Check sheet for the modelled part. Datum: model origin and axes. Units: mm. Face numbers are marked on the shaded views. A direction names the side the tool comes from. Round coordinates to 2 decimals unless told otherwise and drop trailing zeros. Write each loop counter-clockwise with the first axis right and the second up, starting at its lowest first coordinate (ties: lowest second). Pieces come first, ordered by that corner, then holes. Notation, with made-up numbers: (22.25, 81) - (79.25, 81) arc R9 cw to (79.25, 85) - close; hole circle Ø7 at (-29.75, 13). An arc over 180 degrees is marked (long way). Use one line per item in the form item = value. Start each with the question number.
1) Section check C-C (z = 8). Record the boundary of the cut face in (x, y), then the cut area to 3 significant figures.
2) Section check A-A (x = -32.5). Record the boundary of the cut face in (y, z).
3) Set-up check for the marked faces 1, 2 and 3: record each of +Z, -Z, +X, -X, +Y, -Y from which the full face is reachable in a straight line by a thin tool's end or side.
4) Gauge pin test, flat ends, axial feed: P1, Ø4.5, axis at x = 29.5, z = -2.5, coming from the +Y side; P2, Ø14, axis at y = 22, z = 2, coming from the +X side; P3, Ø6, axis at x = -32.5, z = 0, coming from the +Y side; P4, Ø7, axis at y = 2.5, z = -3, coming from the -X side. Record the tip position at first contact, or that the pin passes through.
5) Draft check along X on the marked faces 4, 5 and 6. Enter one of: +X half, -X half, draft (parallel to the pull), parting line (faces both ways), or undercut.
6) Section check B-B (y = 0). Record the boundary of the cut face in (x, z).
7) Scan lines: probe 1 along X at (y, z) = (22, -1.25); probe 2 along Z at (x, y) = (-32.5, -65.5); probe 3 along X at (y, z) = (0, -9.5). Record each from-to range of solid material in increasing order.
8) Section check D-D (z = 0). Record the boundary of the cut face in (x, y), then the cut area to 3 significant figures.
from build123d import *

# Parameters (mm, degrees)
EXTRUDE_1_DEPTH     = 12
SKETCH_2_R          = 3.25
CUT_EXTRUDE_1_DEPTH = 95.704804524


with BuildPart() as part:
    # Sketch 1 → Extrude 1 (new, symmetric)
    with BuildSketch(Plane.XY):
        with BuildLine():
            Line((-40, -70), (40, -70))
            Line((40, -70), (40, -55))
            Line((40, -55), (25, -55))
            Line((25, -55), (25, 30))
            Line((25, 30), (1, 30))
            Line((1, 30), (1, 12.459935794))
            ThreePointArc((1, 12.459935794), (0, -12.5), (-1, 12.459935794))
            Line((-1, 12.459935794), (-1, 30))
            Line((-1, 30), (-25, 30))
            Line((-25, 30), (-25, -55))
            Line((-25, -55), (-40, -55))
            Line((-40, -55), (-40, -70))
        make_face()
    extrude(amount=EXTRUDE_1_DEPTH, both=True)

    # Sketch 2 → Cut-Extrude 1 (cut, through all)
    with BuildSketch(Plane(origin=(0, -55, 0), x_dir=(1, 0, 0), z_dir=(0, 1, 0))):
        with Locations(Location((-32.5, 0, 0), (0, 0, 180))):
            Circle(SKETCH_2_R)
        with Locations((32.5, 0)):
            Circle(SKETCH_2_R)
    extrude(amount=-CUT_EXTRUDE_1_DEPTH, mode=Mode.SUBTRACT)


solid = part.part
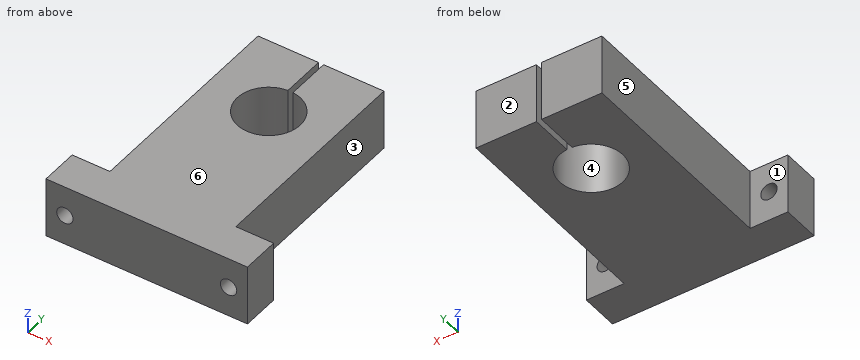
Results are:
q1.outline = (-40, -70) - (40, -70) - (40, -55) - (25, -55) - (25, 30) - (1, 30) - (1, 12.46) arc R12.5 cw (long way) to (-1, 12.46) - (-1, 30) - (-25, 30) - (-25, -55) - (-40, -55) - close
q1.area = 4,920 mm²
q2.outline = (-70, -12) - (-55, -12) - (-55, -3.25) - (-70, -3.25) - close; (-70, 3.25) - (-55, 3.25) - (-55, 12) - (-70, 12) - close
q3.face_1 = +Z, -Z, -X, +Y
q3.face_2 = +Z, -Z, +X, -X, +Y
q3.face_3 = +Z, -Z, +X, +Y
q4.P1 = -55
q4.P2 = 25
q4.P3 = through
q4.P4 = -25
q5.face_4 = undercut
q5.face_5 = -X half
q5.face_6 = draft
q6.outline = (-25, -12) - (-12.5, -12) - (-12.5, 12) - (-25, 12) - close; (12.5, -12) - (25, -12) - (25, 12) - (12.5, 12) - close
q7.probe_1 = -25 to -1, 1 to 25
q7.probe_2 = -12 to -3.25, 3.25 to 12
q7.probe_3 = -25 to -12.5, 12.5 to 25
q8.outline = (-40, -70) - (-35.75, -70) - (-35.75, -55) - (-40, -55) - close; (-29.25, -70) - (29.25, -70) - (29.25, -55) - (25, -55) - (25, 30) - (1, 30) - (1, 12.46) arc R12.5 cw (long way) to (-1, 12.46) - (-1, 30) - (-25, 30) - (-25, -55) - (-29.25, -55) - close; (35.75, -70) - (40, -70) - (40, -55) - (35.75, -55) - close
q8.area = 4,730 mm²
